Design review of the part built by this model. Coordinates are the model's own, in mm. Coordinates: 2 decimals unless noted, no trailing zeros. Write each loop counter-clockwise with the first axis right and the second up, starting at its lowest first coordinate (ties: lowest second). Pieces come first, ordered by that corner, then holes. Notation, with made-up numbers: M -25.75,1 L 33.25,1 A38 cw 33.25,39 Z; hole C -24,4.5 d8. An arc over 180 degrees is marked long. Write each question's results on one line, items separated by ' | '. Start each with the question number.
```python
from build123d import *

# Parameters (mm, degrees)
SKETCH1_W           = 15.3
SKETCH1_H           = 10.2
BOSS_EXTRUDE1_DEPTH = 0.769999908
SKETCH2_W           = 13.9
SKETCH2_H           = 8.7
BOSS_EXTRUDE2_DEPTH = 0.165
WRAP1_START         = -0.0254
WRAP1_OUTLINE_W     = 11.25
WRAP1_OUTLINE_H     = 5.986
WRAP1_DEPTH         = 0.0254


# Read off the part's stored shape, not the designer's step: Wrap1
with BuildPart() as part:
    # Sketch1 → Boss-Extrude1 (new body)
    with BuildSketch(Plane.XY):
        with Locations((-81.255128869, 18.226331852)):
            Rectangle(SKETCH1_W, SKETCH1_H)
    extrude(amount=BOSS_EXTRUDE1_DEPTH)

    # Sketch2 → Boss-Extrude2 (add)
    with BuildSketch(Plane.XY.offset(0.769999908)):
        with Locations((-81.455128869, 18.676331852)):
            Rectangle(SKETCH2_W, SKETCH2_H)
    extrude(amount=BOSS_EXTRUDE2_DEPTH)

    # Wrap1 outline → Wrap1 (cut)
    with BuildSketch(Plane.XY.offset(0.934999908).offset(WRAP1_START)):
        with Locations((-81.255128869, 18.876331852)):
            Rectangle(WRAP1_OUTLINE_W, WRAP1_OUTLINE_H)
    extrude(amount=WRAP1_DEPTH, mode=Mode.SUBTRACT)


solid = part.part
```
Item 1: We need section A-A on x = -79.25. State the section outline as (y, z) points (3 decimals).
Item 2: Draft analysis for pull direction Y (two halves, no side actions). For faces 1 (the flat face through (-81, 14, 0.77)), 2 (the flat face through (-81, 19, 0.91)), state which applies: released by +Y, released by -Y, zero draft, split by the parting line, or undercut.
Item 3: We need section D-D on y = 14. State the section outline as (x, z) points.
Item 4: We need section B-B on y = 15.5. State the section outline as (x, z) points (3 decimals).
Item 5: Insertion check: pin 1 Ø2 at (x, y) = (-84.5, 19) entering from +Z. The pin has a flat end and moves straight along its axis. Give the tip position at first contact, or say it passes through.
Item 6: We need section C-C on y = 18.5. State the section outline as (x, z) points (3 decimals), then the cut area to 3 significant figures.
Item 7: Wall thickness on L1, parallel to Z at x = -83.5, y = 14; L2, parallel to Z at x = -86.5, y = 17.5; L3, parallel to Y at x = -83.75, z = 0.8: over which ranges is each line inside the solid? List them lowest first.
Answer:
1) outline: M 13.126,0 L 23.326,0 L 23.326,0.77 L 23.026,0.77 L 23.026,0.935 L 21.869,0.935 L 21.869,0.91 L 15.883,0.91 L 15.883,0.935 L 14.326,0.935 L 14.326,0.77 L 13.126,0.77 Z
2) face 1: zero draft | face 2: undercut
3) outline: M -88.91,0 L -73.61,0 L -73.61,0.77 L -88.91,0.77 Z
4) outline: M -88.905,0 L -73.605,0 L -73.605,0.77 L -74.505,0.77 L -74.505,0.935 L -88.405,0.935 L -88.405,0.77 L -88.905,0.77 Z
5) pin 1: stops at z = 0.91
6) outline: M -88.905,0 L -73.605,0 L -73.605,0.77 L -74.505,0.77 L -74.505,0.935 L -75.63,0.935 L -75.63,0.91 L -86.88,0.91 L -86.88,0.935 L -88.405,0.935 L -88.405,0.77 L -88.905,0.77 Z | area: 13.8 mm^2
7) L1: z = 0 to 0.77 | L2: z = 0 to 0.91 | L3: y = 14.33 to 23.03
